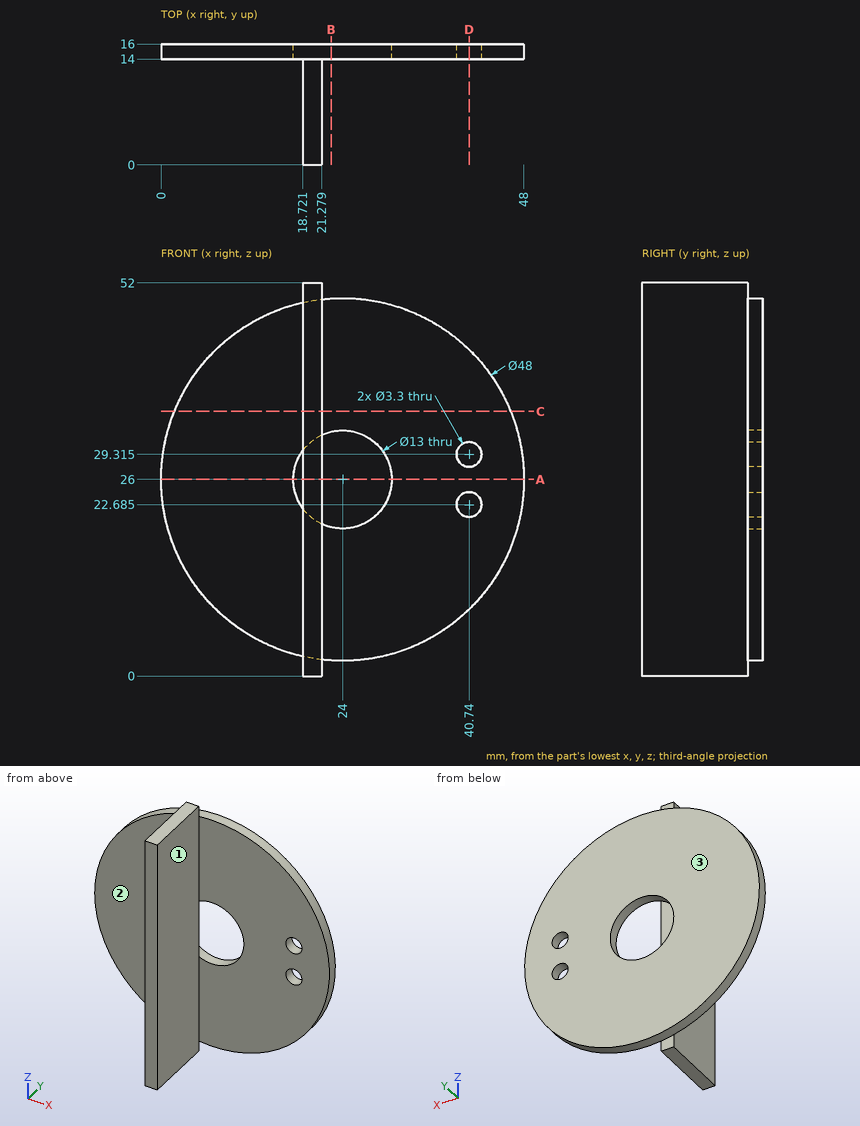
For this review, use the dimensioned drawing (mm, ordinates from the lowest corner) and the shaded views. A direction names the side the tool comes from. Round coordinates to 2 decimals unless told otherwise and drop trailing zeros. Write each loop counter-clockwise with the first axis right and the second up, starting at its lowest first coordinate (ties: lowest second). Pieces come first, ordered by that corner, then holes. Notation, with made-up numbers: M 21.5,-3.5 L 45.5,-3.5 A8 ccw 45.5,2.5 Z; hole C 19.25,53 d7. An arc over 180 degrees is marked long. Use CSV: the item, a comma, the result in double quotes. Start each with the question number.
(1) For line 1 along Z through (x, y) = (24, 15.3); line 2 along Z through (x, y) = (40.74, 14.5) (1 decimal); line 3 along X through (y, z) = (4, 17.5), list the stretches that pass through material, from the lowest coordinate up.
(2) We need section C-C, the plane z = 35. State the section outline as (x, y) points, then the cut area to 3 significant figures.
(3) Clearance check with flat-ended pins moving along their axes: P1, Ø8, axis at y = 9, z = 26, coming from the +X side; P2, Ø1.5, axis at y = 11.5, z = 31.5, coming from the -X side; P3, Ø8, axis at x = 28.5, z = 32, coming from the -Y side; P4, Ø3, axis at x = 19.5, z = 1, coming from the +Y side. State where each tip first meets the part, or that it passes through.
(4) We need section A-A, the plane z = 26. State the section outline as (x, y) points, then the cut area to 3 significant figures.
(5) Tool access review of the marked faces 1, 2 and 3: name each direction out of +Z, -Z, +X, -X, +Y, -Y from which nothing blocks a thin tool from reaching the whole face with its end or side.
(6) We need section B-B, the plane x = 22.5. State the section outline as (y, z) points (1 decimal).
(7) We need section D-D, the plane x = 40.74. State the section outline as (y, z) points (1 decimal), then the cut area to 3 significant figures.
Findings:
1,line 1,"2 to 19.5, 32.5 to 50"
1,line 2,"8.8 to 21, 24.3 to 27.7, 31 to 43.2"
1,line 3,"18.72 to 21.28"
2,outline,"M 1.75,14 L 18.72,14 L 18.72,0 L 21.28,0 L 21.28,14 L 46.25,14 L 46.25,16 L 1.75,16 Z"
2,area,"125 mm^2"
3,P1,"x = 21.28"
3,P2,"x = 18.72"
3,P3,"y = 14"
3,P4,"y = 16"
4,outline,"M 0,14 L 17.5,14 L 17.5,16 L 0,16 Z; M 18.72,0 L 21.28,0 L 21.28,14 L 18.72,14 Z; M 30.5,14 L 48,14 L 48,16 L 30.5,16 Z"
4,area,"106 mm^2"
5,face 1,"+Z, -Z, +X, -Y"
5,face 2,"+Z, -Z, -X, -Y"
5,face 3,"+Z, -Z, +X, -X, +Y"
6,outline,"M 14,2 L 16,2 L 16,19.7 L 14,19.7 Z; M 14,32.3 L 16,32.3 L 16,50 L 14,50 Z"
7,outline,"M 14,8.8 L 16,8.8 L 16,21 L 14,21 Z; M 14,24.3 L 16,24.3 L 16,27.7 L 14,27.7 Z; M 14,31 L 16,31 L 16,43.2 L 14,43.2 Z"
7,area,"55.6 mm^2"
